```python
from build123d import *

# Parameters (mm, degrees)
SKETCH3_R                = 2.5527
BOSS_EXTRUDE1_DEPTH      = 85.725
BOSS_EXTRUDE1_DEPTH_BACK = 85.725


with BuildPart() as part:
    # Sketch3 → Boss-Extrude1 (new body, two sides)
    with BuildSketch(Plane(origin=(0, 0, 0), x_dir=(0, 0, -1), z_dir=(1, 0, 0))) as boss_extrude1_sk:
        with BuildLine():
            Line((-10.668, 12.7), (-3.2385, 12.7))
            Line((-3.2385, 12.7), (-3.2385, 10.3632))
            Line((-3.2385, 10.3632), (-8.800635435, 10.3632))
            Line((-8.800635435, 10.3632), (-3.187235669, 4.749800235))
            Line((-3.187235669, 4.749800235), (3.187235669, 4.749800235))
            Line((3.187235669, 4.749800235), (8.800635435, 10.3632))
            Line((8.800635435, 10.3632), (3.2385, 10.3632))
            Line((3.2385, 10.3632), (3.2385, 12.7))
            Line((3.2385, 12.7), (10.668, 12.7))
            ThreePointArc((10.668, 12.7), (12.104840979, 12.104840979), (12.7, 10.668))
            Line((12.7, 10.668), (12.7, 3.2385))
            Line((12.7, 3.2385), (10.3632, 3.2385))
            Line((10.3632, 3.2385), (10.3632, 8.800635435))
            Line((10.3632, 8.800635435), (4.749800235, 3.187235669))
            Line((4.749800235, 3.187235669), (4.749800235, -3.187235669))
            Line((4.749800235, -3.187235669), (10.3632, -8.800635435))
            Line((10.3632, -8.800635435), (10.3632, -3.2385))
            Line((10.3632, -3.2385), (12.7, -3.2385))
            Line((12.7, -3.2385), (12.7, -10.668))
            ThreePointArc((12.7, -10.668), (12.104840979, -12.104840979), (10.668, -12.7))
            Line((10.668, -12.7), (6.35, -12.7))
            ThreePointArc((6.35, -12.7), (-7.120384182, -7.120384182), (-12.7, 6.35))
            Line((-12.7, 6.35), (-12.7, 10.668))
            ThreePointArc((-12.7, 10.668), (-12.104840979, 12.104840979), (-10.668, 12.7))
        make_face()
        Circle(SKETCH3_R, mode=Mode.SUBTRACT)
        with BuildLine():
            Line((2.485198871, -4.047763436), (8.003751298, -9.566315863))
            ThreePointArc((8.003751298, -9.566315863), (-4.965122713, -4.965122713), (-9.566315863, 8.003751298))
            Line((-9.566315863, 8.003751298), (-4.047763436, 2.485198871))
            ThreePointArc((-4.047763436, 2.485198871), (-3.358615955, -3.358615955), (2.485198871, -4.047763436))
        make_face(mode=Mode.SUBTRACT)
    extrude(amount=BOSS_EXTRUDE1_DEPTH)
    extrude(boss_extrude1_sk.sketch, amount=-BOSS_EXTRUDE1_DEPTH_BACK)


solid = part.part
```
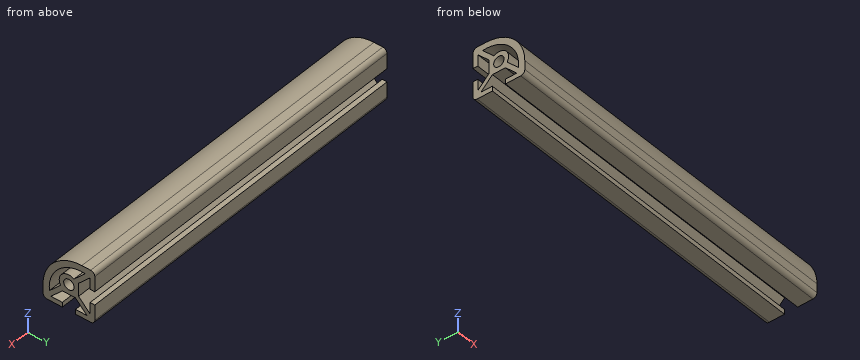
Work out the finished part from the listing and answer in its coordinate system (mm). Coordinates: 2 decimals unless noted, no trailing zeros. Loops run counter-clockwise (first coordinate to the right, second up) from the corner with the lowest first, then second, coordinate; pieces in that order, holes last.
1) Consider probe 1 along Z at (x, y) = (24.5, -2); probe 2 along Y at (x, z) = (-35.5, -4); probe 3 along Z at (x, y) = (15.5, -6). Determine where each line is inside the solid, lowest interval first.
Results:
probe 1: z = -4.75 to -1.59, 1.59 to 4.31, 7.3 to 10.77
probe 2: y = -12.55 to -9.48, -5.56 to 5.56, 10.36 to 12.7
probe 3: z = -12.7 to -10.36, -7.56 to -4.44, 3.83 to 8.15
2) Section B-B (z = 0) is taken. Give the vertices of the cut face in (x, y) (3 decimals).
Results:
outline: (-85.725, -11.611) - (85.725, -11.611) - (85.725, -8.338) - (-85.725, -8.338) - close; (-85.725, -4.75) - (85.725, -4.75) - (85.725, -2.553) - (-85.725, -2.553) - close; (-85.725, 2.553) - (85.725, 2.553) - (85.725, 4.75) - (-85.725, 4.75) - close
3) Section C-C (y = 0) is taken. Give the vertices of the cut face in (x, z) (3 decimals).
Results:
outline: (-85.725, -4.75) - (85.725, -4.75) - (85.725, -2.553) - (-85.725, -2.553) - close; (-85.725, 2.553) - (85.725, 2.553) - (85.725, 4.75) - (-85.725, 4.75) - close; (-85.725, 8.338) - (85.725, 8.338) - (85.725, 11.611) - (-85.725, 11.611) - close
4) Section A-A (x = -39) is taken. Give the number of separate pieces and of enclosed holes in the cut face, plus the area to 3 significant figures.
Results:
separate pieces: 1
enclosed holes: 2
area: 302 mm2
5) Flat-ended cylindrical pins translate along their axes: pin 1 (3 mm diameter, centred on x = 0, z = 6.5, fed in from -Y); pin 2 (5 mm diameter, centred on x = -52.5, z = 1.5, fed in from -Y); pin 3 (5 mm diameter, centred on x = -6.5, y = 0.5, fed in from -Z). Find the tip coordinate at first contact, or state that the pin passes through.
Results:
pin 1: stops at y = -8.95
pin 2: stops at y = -11.93
pin 3: stops at z = -4.75
